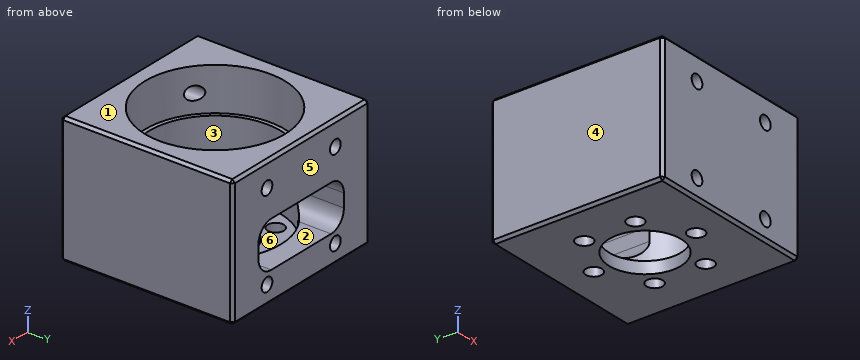
```python
from build123d import *

# Parameters (mm, degrees)
SKETCH_1_R               = 16
SKETCH_1_R_2             = 6.65
EXTRUDE_1_DEPTH          = 24
SKETCH_3_R               = 1.5
CUT_EXTRUDE_2_DEPTH      = 33.984845005
PATTERN_CIRCULAR_1_COUNT = 6
EXTRUDE_START            = -24
EXTRUDE_2_DEPTH          = 24
SKETCH_7_R               = 13
CUT_EXTRUDE_3_DEPTH      = 21.8
EXTRUDE_START_2          = 13.8
SKETCH_15_R              = 13
SKETCH_15_R_2            = 12.25
EXTRUDE_4_DEPTH          = 13.8
SKETCH_11_W              = 20
SKETCH_11_H              = 8.5
CUT_EXTRUDE_4_DEPTH      = 10
FILLET_1_R               = 3
SKETCH_12_R              = 1
CUT_EXTRUDE_5_DEPTH      = 44.081318457
HOLE_WIZARD_M3_1_D       = 2.5
CHAMFER_1_SIZE           = 0.5


with BuildPart() as part:
    # 草图1 → 凸台-拉伸1 (new body)
    with BuildSketch(Plane.XY):
        Circle(SKETCH_1_R)
        Circle(SKETCH_1_R_2, mode=Mode.SUBTRACT)
    extrude(amount=EXTRUDE_1_DEPTH)

    # 草图3 → 切除-拉伸2 (cut, through all)
    with BuildSketch(Plane(origin=(0, 0, 0), x_dir=(-1, 0, 0), z_dir=(0, 0, -1))):
        with Locations((0, 9.5)):
            Circle(SKETCH_3_R)
    cut_extrude_2 = extrude(amount=-CUT_EXTRUDE_2_DEPTH, mode=Mode.SUBTRACT)

    # 阵列(圆周)1: 切除-拉伸2 ×6 about axis
    pattern_circular_1_axis = Axis((0, 0, 0), (0, 0, 1))
    for i in range(1, PATTERN_CIRCULAR_1_COUNT):
        add(cut_extrude_2.rotate(pattern_circular_1_axis, i * 360 / PATTERN_CIRCULAR_1_COUNT), mode=Mode.SUBTRACT)

    # 草图4 → 凸台-拉伸2 (add)
    with BuildSketch(Plane.XY.offset(24).offset(EXTRUDE_START)):
        with BuildLine():
            ThreePointArc((16, 0), (11.313708518, -11.31370848), (5.5e-08, -16))
            Line((5.5e-08, -16), (16, -16))
            Line((16, -16), (16, 0))
        make_face()
        with BuildLine():
            ThreePointArc((5.5e-08, -16), (-11.31370848, -11.313708518), (-16, 0))
            Line((-16, 0), (-16, -16))
            Line((-16, -16), (5.5e-08, -16))
        make_face()
        with BuildLine():
            Line((-16, 16), (-16, 0))
            ThreePointArc((-16, 0), (-11.313708518, 11.31370848), (-5.5e-08, 16))
            Line((-5.5e-08, 16), (-16, 16))
        make_face()
        with BuildLine():
            Line((16, 16), (-5.5e-08, 16))
            ThreePointArc((-5.5e-08, 16), (11.31370848, 11.313708518), (16, 0))
            Line((16, 0), (16, 16))
        make_face()
    extrude(amount=EXTRUDE_2_DEPTH)

    # 草图7 → 切除-拉伸3 (cut)
    with BuildSketch(Plane.XY.offset(24)):
        Circle(SKETCH_7_R)
    extrude(amount=-CUT_EXTRUDE_3_DEPTH, mode=Mode.SUBTRACT)

    # 草图15 → 凸台-拉伸4 (add)
    with BuildSketch(Plane.XY.offset(2.2).offset(EXTRUDE_START_2)):
        Circle(SKETCH_15_R)
        Circle(SKETCH_15_R_2, mode=Mode.SUBTRACT)
    extrude(amount=-EXTRUDE_4_DEPTH)

    # 草图11 → 切除-拉伸4 (cut)
    with BuildSketch(Plane(origin=(0, 16, 0), x_dir=(1, 0, 0), z_dir=(0, 1, 0))):
        with Locations((0, -9.75)):
            Rectangle(SKETCH_11_W, SKETCH_11_H)
    extrude(amount=-CUT_EXTRUDE_4_DEPTH, mode=Mode.SUBTRACT)

    # 圆角1
    fillet_1_edges = [part.edges().sort_by_distance(p)[0] for p in [
        (10, 11.537742925, 5.5),
        (10, 11.537742925, 14),
        (-10, 11.537742925, 14),
        (-10, 11.537742925, 5.5),
    ]]
    fillet(fillet_1_edges, radius=FILLET_1_R)

    # 草图12 → 切除-拉伸5 (cut, through all)
    with BuildSketch(Plane(origin=(0, 16, 0), x_dir=(1, 0, 0), z_dir=(0, 1, 0))):
        with Locations(Location((8, -3.5, 0), (0, 0, 180))):
            Circle(SKETCH_12_R)
        with Locations(Location((8, -19.5, 0), (0, 0, 180))):
            Circle(SKETCH_12_R)
        with Locations(Location((-8, -3.5, 0), (0, 0, 180))):
            Circle(SKETCH_12_R)
        with Locations(Location((-8, -19.5, 0), (0, 0, 180))):
            Circle(SKETCH_12_R)
    extrude(amount=-CUT_EXTRUDE_5_DEPTH, mode=Mode.SUBTRACT)

    # M3 螺纹孔1 (through all)
    with Locations(Plane(origin=(0, 16, 0), x_dir=(1, 0, 0), z_dir=(0, 1, 0))):
        with Locations((8, -3.5), (-8, -3.5), (-8, -19.5), (8, -19.5)):
            Hole(HOLE_WIZARD_M3_1_D / 2)

    # 倒角1
    chamfer_1_edges = [part.edges().sort_by_distance(p)[0] for p in [
        (0, -16, 24),
        (16, -16, 12),
        (16, 0, 0),
        (16, 0, 24),
        (0, -16, 0),
        (-16, -16, 12),
        (-16, 0, 24),
        (-16, 0, 0),
        (0, 16, 0),
        (-16, 16, 12),
        (0, 16, 24),
        (16, 16, 12),
    ]]
    chamfer(chamfer_1_edges, length=CHAMFER_1_SIZE)


solid = part.part
```
Geometry check sheet. Reference: the model listing, model coordinates, mm. Face numbers are marked on the shaded views. A direction names the side the tool comes from. Give positions to 0.01 mm unless a question says otherwise; leave off trailing zeros. Order: outer loops, then holes, each group sorted by start corner. A loop starts at its lowest first (then second) coordinate and runs counter-clockwise, first axis right, second up.
1. Release check for a two-part mould opening along Y. For the marked faces 4, 5 and 6 record: pulls with the +Y half, pulls with the -Y half, needs draft (parallel to the pull), parting line crosses it, or undercut.
2. Section check B-B, the plane z = 3. Enter the section's corners in (x, y), and give its area (3 significant figures).
3. Section check D-D, the plane y = -14. Enter the section's corners in (x, z).
4. Section check A-A, the plane y = 0. Enter the section's corners in (x, z), and give its area (3 significant figures).
5. Gauge pin test, flat ends, axial feed: pin 1 Ø2.5 at (x, y) = (0, -9.5) entering from -Z; pin 2 Ø4 at (x, y) = (8.23, 4.75) entering from +Z. Record the tip position at first contact, or that the pin passes through.
6. Access from +Z, -Z, +X, -X, +Y, -Y to the whole of each face (thin tool, end or side, straight path). Record for the marked faces 1, 2 and 3.
7. Thickness scan on L1, parallel to Y at x = 0, z = 0.65; L2, parallel to Z at x = -8, y = -11; L3, parallel to Z at x = -8, y = -10. Record the ranges inside material, lowest first.
8. Section check C-C, the plane y = 14. Enter the section's corners in (x, z).
Values follow:
1. face 4: needs draft
1. face 5: pulls with the +Y half
1. face 6: undercut
2. outline: (-16, -15.5) - (-15.5, -16) - (-9.15, -16) - (-9.15, -8.15) arc R12.25 cw to (-9.15, 8.15) - (-9.15, 16) - (-15.5, 16) - (-16, 15.5) - close; (-6.85, -16) - (6.85, -16) - (6.85, -10.15) arc R12.25 cw to (-6.85, -10.15) - close; (-6.85, 10.15) arc R12.25 cw to (6.85, 10.15) - (6.85, 16) - (-6.85, 16) - close; (9.15, -16) - (15.5, -16) - (16, -15.5) - (16, 15.5) - (15.5, 16) - (9.15, 16) - (9.15, 8.15) arc R12.25 cw to (9.15, -8.15) - close
2. area: 490 mm2
3. outline: (-16, 0.5) - (-15.5, 0) - (15.5, 0) - (16, 0.5) - (16, 23.5) - (15.5, 24) - (-15.5, 24) - (-16, 23.5) - close; hole circle Ø2.5 at (-8, 3.5); hole circle Ø2.5 at (-8, 19.5); hole circle Ø2.5 at (8, 3.5); hole circle Ø2.5 at (8, 19.5)
4. outline: (-16, 0.5) - (-15.5, 0) - (-6.65, 0) - (-6.65, 2.2) - (-12.25, 2.2) - (-12.25, 16) - (-13, 16) - (-13, 24) - (-15.5, 24) - (-16, 23.5) - close; (6.65, 0) - (15.5, 0) - (16, 0.5) - (16, 23.5) - (15.5, 24) - (13, 24) - (13, 16) - (12.25, 16) - (12.25, 2.2) - (6.65, 2.2) - close
4. area: 192 mm2
5. pin 1: passes through
5. pin 2: stops at z = 2.2
6. face 1: +Z, +X, -X, +Y, -Y
6. face 2: +Y
6. face 3: +Z
7. L1: y = -16 to -11, -8 to -6.65, 6.65 to 8, 11 to 16
7. L2: z = 0 to 2.25, 4.75 to 18.25, 20.75 to 24
7. L3: z = 0 to 2.25, 4.75 to 16
8. outline: (-16, 0.5) - (-15.5, 0) - (15.5, 0) - (16, 0.5) - (16, 23.5) - (15.5, 24) - (-15.5, 24) - (-16, 23.5) - close; hole (-10, 8.5) arc R3 ccw to (-7, 5.5) - (7, 5.5) arc R3 ccw to (10, 8.5) - (10, 11) arc R3 ccw to (7, 14) - (-7, 14) arc R3 ccw to (-10, 11) - close; hole circle Ø2.5 at (-8, 3.5); hole circle Ø2.5 at (-8, 19.5); hole circle Ø2.5 at (8, 3.5); hole circle Ø2.5 at (8, 19.5)
